Geometry check sheet. Reference: the model listing, model coordinates, mm. Round coordinates to 2 decimals unless told otherwise and drop trailing zeros. Write each loop counter-clockwise with the first axis right and the second up, starting at its lowest first coordinate (ties: lowest second). Pieces come first, ordered by that corner, then holes. Notation, with made-up numbers: (1.25, 49) -> (52.25, 49) arc R12 ccw to (52.25, 56) -> close; hole circle Ø9 at (-26.5, 53). An arc over 180 degrees is marked (long way). Use a Markdown table: item, result.
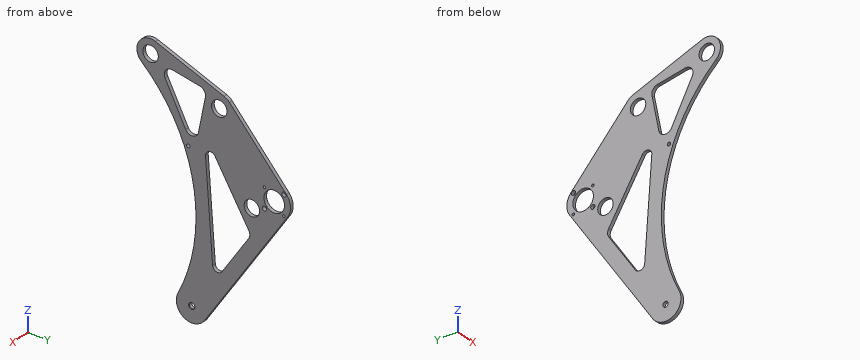
```python
from build123d import *

# Parameters (mm, degrees)
BOSS_EXTRUDE1_DEPTH               = 6.35
CUT_EXTRUDE1_REACH                = 8.35
SKETCH3_R                         = 14.2875
SKETCH3_R_2                       = 19.05
SKETCH3_R_3                       = 2.413
SKETCH3_R_4                       = 3.96875
F_3_8_CLEARANCE_HOLE2_D           = 9.8044
F_3_8_CLEARANCE_HOLE2_CSINK_D     = 11.58748
F_3_8_CLEARANCE_HOLE2_CSINK_ANGLE = 90
F_1_4_0_2500_DOWEL_HOLE2_D        = 6.35
CUT_EXTRUDE2_DEPTH                = 7.35


with BuildPart() as part:
    # Sketch2 → Boss-Extrude1 (new body)
    with BuildSketch(Plane(origin=(0, 0, 0), x_dir=(0, 0, -1), z_dir=(1, 0, 0))):
        with BuildLine():
            Line((-420.65776111, -67.281464584), (-373.03276111, 59.718535416))
            ThreePointArc((-373.03276111, 59.718535416), (-370.217283815, 65.136422477), (-366.190217158, 69.725882876))
            Line((-366.190217158, 69.725882876), (-248.716507876, 174.874485915))
            ThreePointArc((-248.716507876, 174.874485915), (-230.65414247, 182.492472563), (-211.724122614, 177.399623371))
            Line((-211.724122614, 177.399623371), (15.987673313, 23.68385372))
            ThreePointArc((15.987673313, 23.68385372), (24.617664495, -14.508660165), (-12.975284095, -25.459234624))
            ThreePointArc((-12.975284095, -25.459234624), (-206.983757432, 2.660555148), (-377.990639572, -93.186492612))
            ThreePointArc((-377.990639572, -93.186492612), (-410.057040874, -97.911605155), (-420.65776111, -67.281464584))
        make_face()
    extrude(amount=BOSS_EXTRUDE1_DEPTH)

    # Sketch3 → Cut-Extrude1 (cut, up to next)
    with BuildSketch(Plane(origin=(6.35, 0, 0), x_dir=(0, 0, -1), z_dir=(1, 0, 0)), mode=Mode.PRIVATE) as cut_extrude1_sk1:
        with Locations((-203.2, 111.125)):
            Circle(SKETCH3_R)
    cut_extrude1_tool1 = extrude(cut_extrude1_sk1.sketch, amount=-CUT_EXTRUDE1_REACH, mode=Mode.PRIVATE) & part.part
    add(cut_extrude1_tool1.solids().sort_by_distance((6.35, 111.125, 203.2))[0], mode=Mode.SUBTRACT)
    # Sketch3 → Cut-Extrude1 (cut, up to next)
    with BuildSketch(Plane(origin=(6.35, 0, 0), x_dir=(0, 0, -1), z_dir=(1, 0, 0)), mode=Mode.PRIVATE) as cut_extrude1_sk2:
        with Locations((-349.25, 50.8)):
            Circle(SKETCH3_R)
    cut_extrude1_tool2 = extrude(cut_extrude1_sk2.sketch, amount=-CUT_EXTRUDE1_REACH, mode=Mode.PRIVATE) & part.part
    add(cut_extrude1_tool2.solids().sort_by_distance((6.35, 50.8, 349.25))[0], mode=Mode.SUBTRACT)
    # Sketch3 → Cut-Extrude1 (cut, up to next)
    with BuildSketch(Plane(origin=(6.35, 0, 0), x_dir=(0, 0, -1), z_dir=(1, 0, 0)), mode=Mode.PRIVATE) as cut_extrude1_sk3:
        with Locations((-396.875, -76.2)):
            Circle(SKETCH3_R)
    cut_extrude1_tool3 = extrude(cut_extrude1_sk3.sketch, amount=-CUT_EXTRUDE1_REACH, mode=Mode.PRIVATE) & part.part
    add(cut_extrude1_tool3.solids().sort_by_distance((6.35, -76.2, 396.875))[0], mode=Mode.SUBTRACT)
    # Sketch3 → Cut-Extrude1 (cut, up to next)
    with BuildSketch(Plane(origin=(6.35, 0, 0), x_dir=(0, 0, -1), z_dir=(1, 0, 0)), mode=Mode.PRIVATE) as cut_extrude1_sk4:
        with Locations((-228.6, 152.4)):
            Circle(SKETCH3_R_2)
    cut_extrude1_tool4 = extrude(cut_extrude1_sk4.sketch, amount=-CUT_EXTRUDE1_REACH, mode=Mode.PRIVATE) & part.part
    add(cut_extrude1_tool4.solids().sort_by_distance((6.35, 152.4, 228.6))[0], mode=Mode.SUBTRACT)
    # Sketch3 → Cut-Extrude1 (cut, up to next)
    with BuildSketch(Plane(origin=(6.35, 0, 0), x_dir=(0, 0, -1), z_dir=(1, 0, 0)), mode=Mode.PRIVATE) as cut_extrude1_sk5:
        with Locations((-246.560512242, 134.439487758)):
            Circle(SKETCH3_R_3)
    cut_extrude1_tool5 = extrude(cut_extrude1_sk5.sketch, amount=-CUT_EXTRUDE1_REACH, mode=Mode.PRIVATE) & part.part
    add(cut_extrude1_tool5.solids().sort_by_distance((6.35, 134.439488, 246.560512))[0], mode=Mode.SUBTRACT)
    # Sketch3 → Cut-Extrude1 (cut, up to next)
    with BuildSketch(Plane(origin=(6.35, 0, 0), x_dir=(0, 0, -1), z_dir=(1, 0, 0)), mode=Mode.PRIVATE) as cut_extrude1_sk6:
        with Locations((-210.639487758, 134.439487758)):
            Circle(SKETCH3_R_4)
    cut_extrude1_tool6 = extrude(cut_extrude1_sk6.sketch, amount=-CUT_EXTRUDE1_REACH, mode=Mode.PRIVATE) & part.part
    add(cut_extrude1_tool6.solids().sort_by_distance((6.35, 134.439488, 210.639488))[0], mode=Mode.SUBTRACT)
    # Sketch3 → Cut-Extrude1 (cut, up to next)
    with BuildSketch(Plane(origin=(6.35, 0, 0), x_dir=(0, 0, -1), z_dir=(1, 0, 0)), mode=Mode.PRIVATE) as cut_extrude1_sk7:
        with Locations((-210.639487758, 170.360512242)):
            Circle(SKETCH3_R_3)
    cut_extrude1_tool7 = extrude(cut_extrude1_sk7.sketch, amount=-CUT_EXTRUDE1_REACH, mode=Mode.PRIVATE) & part.part
    add(cut_extrude1_tool7.solids().sort_by_distance((6.35, 170.360512, 210.639488))[0], mode=Mode.SUBTRACT)
    # Sketch3 → Cut-Extrude1 (cut, up to next)
    with BuildSketch(Plane(origin=(6.35, 0, 0), x_dir=(0, 0, -1), z_dir=(1, 0, 0)), mode=Mode.PRIVATE) as cut_extrude1_sk8:
        with Locations((-246.560512242, 170.360512242)):
            Circle(SKETCH3_R_4)
    cut_extrude1_tool8 = extrude(cut_extrude1_sk8.sketch, amount=-CUT_EXTRUDE1_REACH, mode=Mode.PRIVATE) & part.part
    add(cut_extrude1_tool8.solids().sort_by_distance((6.35, 170.360512, 246.560512))[0], mode=Mode.SUBTRACT)

    # 3/8 Clearance Hole2 (through all)
    with Locations(Plane(origin=(6.35, 0, 0), x_dir=(0, 0, -1), z_dir=(1, 0, 0))):
        with Locations((0, 0)):
            CounterSinkHole(F_3_8_CLEARANCE_HOLE2_D / 2, F_3_8_CLEARANCE_HOLE2_CSINK_D / 2, counter_sink_angle=F_3_8_CLEARANCE_HOLE2_CSINK_ANGLE)

    # 1/4 (0.2500) Dowel Hole2 (through all)
    with Locations(Plane(origin=(6.35, 0, 0), x_dir=(0, 0, -1), z_dir=(1, 0, 0))):
        with Locations((-266.7, -6.35)):
            Hole(F_1_4_0_2500_DOWEL_HOLE2_D / 2)

    # Sketch14 → Cut-Extrude2 (cut, through all)
    with BuildSketch(Plane(origin=(6.35, 0, 0), x_dir=(0, 0, -1), z_dir=(1, 0, 0))):
        with BuildLine():
            Line((-365.600411715, -49.359627546), (-292.575411715, -11.259627546))
            ThreePointArc((-292.575411715, -11.259627546), (-285.877370021, 1.794150333), (-295.959325084, 12.453374581))
            Line((-295.959325084, 12.453374581), (-359.459325084, 25.153374581))
            ThreePointArc((-359.459325084, 25.153374581), (-369.058218075, 23.224411423), (-374.432476774, 15.040464395))
            Line((-374.432476774, 15.040464395), (-383.957476774, -35.759535605))
            ThreePointArc((-383.957476774, -35.759535605), (-379.035203223, -48.304573838), (-365.600411715, -49.359627546))
        make_face()
        with BuildLine():
            Line((-77.20752162, 55.949267111), (-149.968519497, 105.066234213))
            ThreePointArc((-149.968519497, 105.066234213), (-156.765517001, 107.236326229), (-163.659929975, 105.39906082))
            Line((-163.659929975, 105.39906082), (-266.47492871, 43.043617869))
            ThreePointArc((-266.47492871, 43.043617869), (-270.608700361, 32.000347521), (-260.837451688, 25.4))
            Line((-260.837451688, 25.4), (-81.838602457, 38.555269198))
            ThreePointArc((-81.838602457, 38.555269198), (-73.332394792, 45.604028308), (-77.20752162, 55.949267111))
        make_face()
    extrude(amount=-CUT_EXTRUDE2_DEPTH, mode=Mode.SUBTRACT)


solid = part.part
```
(1) Thickness scan on line 1 (Y direction, x = 4.25, z = 266.7) (3 decimals); line 2 (Y direction, x = 5.5, z = 202); line 3 (Z direction, x = 5.75, y = 106). Record the ranges inside material, lowest first.
A:
| item | result |
|---|---|
| line 1 | y = -14.883 to -9.525, -3.175 to 26.896, 42.903 to 158.778 |
| line 2 | y = 3.54 to 29.72, 82.15 to 96.89, 125.36 to 170.84 |
| line 3 | z = 105.95 to 151.6, 162.55 to 189.86, 216.54 to 325.66 |
(2) Section check B-B on y = 50.8. Record the cut outline in (x, z).
A:
| item | result |
|---|---|
| outline | (0, 24.18) -> (6.35, 24.18) -> (6.35, 73.42) -> (0, 73.42) -> close; (0, 253.69) -> (6.35, 253.69) -> (6.35, 334.96) -> (0, 334.96) -> close; (0, 363.54) -> (6.35, 363.54) -> (6.35, 376.38) -> (0, 376.38) -> close |
(3) Section check A-A on y = 152.4. Record the cut outline in (x, z), plus the area to 3 significant figures.
A:
| item | result |
|---|---|
| outline | (0, 174.69) -> (6.35, 174.69) -> (6.35, 209.55) -> (0, 209.55) -> close; (0, 247.65) -> (6.35, 247.65) -> (6.35, 273.83) -> (0, 273.83) -> close |
| area | 388 mm2 |
(4) Section check C-C on z = 228.6. Record the cut outline in (x, y), plus the area to 3 significant figures.
A:
| item | result |
|---|---|
| outline | (0, -2.17) -> (6.35, -2.17) -> (6.35, 27.77) -> (0, 27.77) -> close; (0, 66.01) -> (6.35, 66.01) -> (6.35, 133.35) -> (0, 133.35) -> close; (0, 171.45) -> (6.35, 171.45) -> (6.35, 182.56) -> (0, 182.56) -> close |
| area | 688 mm2 |
(5) Section check D-D on x = 2.5. State how many separate pieces and enclosed holes the cut face has, plus the area to 3 significant figures.
A:
| item | result |
|---|---|
| separate pieces | 1 |
| enclosed holes | 12 |
| area | 38,300 mm2 |
(6) Gauge pin test, flat ends, axial feed: pin 1 Ø2 at (x, y) = (4, 61.5) entering from +Z; pin 2 Ø1 at (x, y) = (4, 117) entering from +Z; pin 3 Ø1 at (x, y) = (5.5, 121) entering from -Z; pin 4 Ø3 at (y, z) = (109, 191.5) entering from -X. Record the tip position at first contact, or that the pin passes through.
A:
| item | result |
|---|---|
| pin 1 | stops at z = 372.72 |
| pin 2 | stops at z = 313.93 |
| pin 3 | stops at z = 127.43 |
| pin 4 | passes through |
